Here's how the part is built. I have some questions about the finished solid (model axes, mm). Face numbers are marked on the shaded views. Coordinates: 2 decimals unless noted, no trailing zeros. Write each loop counter-clockwise with the first axis right and the second up, starting at its lowest first coordinate (ties: lowest second). Pieces come first, ordered by that corner, then holes.
(1) For pin 1 Ø5 at (y, z) = (16.5, 11.5) entering from -X; pin 2 Ø3 at (x, y) = (-9.5, 31.5) entering from -Z; pin 3 Ø10 at (x, y) = (-8.5, 0) entering from -Z, each with a flat end and sliding along its axis, tell me the tip position at first contact or that it passes through.
(2) Imagine slicing it at B-B, the plane y = -9.5. List the corners of the cut face in (x, z) for me, plus the area to 3 significant figures.
(3) Imagine slicing it at A-A, the plane x = 0. List the corners of the cut face in (y, z) for me.
(4) Thinking about a two-plate mould opening in Z: for the marked faces 1, 2 and 3, which applies, released by +Z, released by -Z, zero draft, split by the parting line, or undercut?
(5) Please list where these lines run through material, in increasing order: probe 1 along Z at (x, y) = (0, 3); probe 2 along X at (y, z) = (25, 12); probe 3 along X at (y, z) = (31, -16).
(6) Imagine slicing it at C-C, the plane z = 0. State how many separate pieces and enclosed holes the cut face has, plus the area to 3 significant figures.
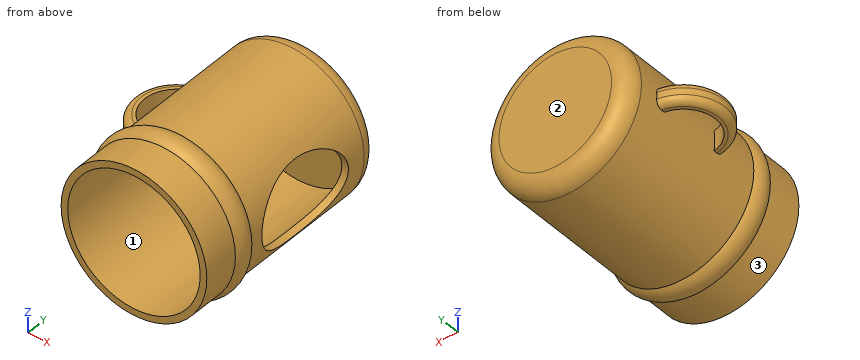
```python
from build123d import *

# Parameters (mm, degrees)
F3_DEPTH = 3
F4_R     = 5
F5_R     = 2
F7_DEPTH = 30


with BuildPart() as f1:
    # F0 (on Top) → F1 (revolve)
    with BuildSketch(Plane.XY):
        Polygon((-20, 43.255373), (0, 43.255373), (0, 45.255373), (-22, 45.255373), (-22, -1.848867), (-22, -8.040607), (-22, -18.744627), (-20, -18.744627), align=None)
        with BuildLine():
            Line((-22, -8.040607), (-22, -1.848867))
            ThreePointArc((-22, -1.848867), (-23.171118, -4.944737), (-22, -8.040607))
        make_face()
    revolve(axis=Axis((0, -2.109665, 0), (0, 1, 0)))

    # F2 (on Top) → F3 (join, symmetric)
    with BuildSketch(Plane.XY):
        with BuildLine():
            ThreePointArc((-20, 12.639232), (-29.646143, 22.148181), (-20, 31.65713))
            Line((-20, 31.65713), (-19.957029, 34.656822))
            ThreePointArc((-19.957029, 34.656822), (-32.646143, 22.148181), (-19.957029, 9.63954))
            Line((-19.957029, 9.63954), (-20, 12.639232))
        make_face()
    extrude(amount=F3_DEPTH, both=True)

    # F4
    f4_edges = [f1.edges().sort_by_distance(p)[0] for p in [
        (22, 45.255373, 0),
    ]]
    fillet(f4_edges, radius=F4_R)

    # F5
    f5_edges = [f1.edges().sort_by_distance(p)[0] for p in [
        (-32.646143, 22.148181, 3),
        (-32.646143, 22.148181, -3),
    ]]
    fillet(f5_edges, radius=F5_R)

    # F6 (on Right) → F7 (cut)
    with BuildSketch(Plane.YZ):
        with BuildLine():
            add(Edge.make_bspline(
                [(34.336799, 0), (34.336799, 19.918584), (10.014392, 9.959292), (-14.308014, 0), (10.014392, -9.959292), (34.336799, -19.918584), (34.336799, 0)],
                knots=[0, 0, 0, 2.094395, 2.094395, 4.18879, 4.18879, 6.283185, 6.283185, 6.283185], degree=2, weights=[1, 0.5, 1, 0.5, 1, 0.5, 1]))
        make_face()
    extrude(amount=F7_DEPTH, mode=Mode.SUBTRACT)


solid = f1.part
```
Recorded:
1. pin 1: stops at x = -20.07
1. pin 2: stops at z = -20.49
1. pin 3: stops at z = -22.42
2. outline: circle Ø44 at (0, 0); hole circle Ø40 at (0, 0)
2. area: 264 mm2
3. outline: (-18.74, -22) - (-8.04, -22) arc R4.68 ccw to (-1.85, -22) - (40.26, -22) arc R5 ccw to (45.26, -17) - (45.26, 17) arc R5 ccw to (40.26, 22) - (-1.85, 22) arc R4.68 ccw to (-8.04, 22) - (-18.74, 22) - (-18.74, 20) - (43.26, 20) - (43.26, -20) - (-18.74, -20) - close
4. face 1: undercut
4. face 2: zero draft
4. face 3: split by the parting line
5. probe 1: z = -22 to -20, 20 to 22
5. probe 2: x = -18.44 to -16, 16 to 18.44
5. probe 3: x = -15.1 to -12, 12 to 15.1
6. separate pieces: 2
6. enclosed holes: 1
6. area: 363 mm2
